```python
from build123d import *

# Parameters (mm, degrees)
BOSS_EXTRUDE1_DEPTH = 12.7
SKETCH1_10_R        = 3.175
SKETCH1_10_R_2      = 6.35
CUT_EXTRUDE3_DEPTH  = 12.7
SKETCH2_W           = 2.54
SKETCH2_H           = 25.4
CUT_EXTRUDE4_DEPTH  = 10.16
SKETCH2_3_W         = 20.32
SKETCH2_3_H         = 3.81
BOSS_EXTRUDE2_DEPTH = 10.16


with BuildPart() as part:
    # Sketch1 → Boss-Extrude1 (new, symmetric)
    with BuildSketch(Plane.XY):
        with BuildLine():
            Line((609.6, 0), (609.6, 25.4))
            Line((609.6, 25.4), (76.2, 25.4))
            ThreePointArc((76.2, 25.4), (63.5, 12.7), (76.2, 0))
            Line((76.2, 0), (609.6, 0))
        make_face()
    extrude(amount=BOSS_EXTRUDE1_DEPTH, both=True)

    # Sketch1<10> → Cut-Extrude3 (cut, symmetric)
    with BuildSketch(Plane.XY):
        with Locations((76.2, 12.7)):
            Circle(SKETCH1_10_R)
        with Locations((139.699994312, 12.7)):
            Circle(SKETCH1_10_R_2)
    extrude(amount=CUT_EXTRUDE3_DEPTH, both=True, mode=Mode.SUBTRACT)

    # Sketch2 → Cut-Extrude4 (cut)
    with BuildSketch(Plane(origin=(609.6, 0, 0), x_dir=(0, 0, -1), z_dir=(1, 0, 0))):
        with Locations((-11.43, 12.7)):
            Rectangle(SKETCH2_W, SKETCH2_H)
        with Locations((11.43, 12.7)):
            Rectangle(SKETCH2_W, SKETCH2_H)
    extrude(amount=-CUT_EXTRUDE4_DEPTH, mode=Mode.SUBTRACT)

    # Sketch2<3> → Boss-Extrude2 (add)
    with BuildSketch(Plane(origin=(609.6, 0, 0), x_dir=(0, 0, -1), z_dir=(1, 0, 0))):
        with Locations((0, 27.305)):
            Rectangle(SKETCH2_3_W, SKETCH2_3_H)
        with Locations((0, -1.905)):
            Rectangle(SKETCH2_3_W, SKETCH2_3_H)
    extrude(amount=-BOSS_EXTRUDE2_DEPTH)


solid = part.part
```
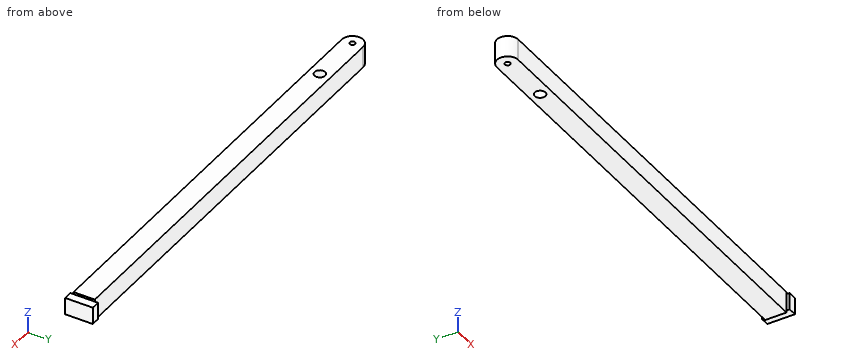
Here's how the part is built. I have some questions about the finished solid (model axes, mm). Give positions to 0.01 mm unless a question says otherwise; leave off trailing zeros. Write each loop counter-clockwise with the first axis right and the second up, starting at its lowest first coordinate (ties: lowest second). Pieces come first, ordered by that corner, then holes. Notation, with made-up numbers: M 0,-1.75 L 10,-1.75 A19 ccw 10,11.25 Z; hole C -39.5,41.25 d9. An arc over 180 degrees is marked long. Put each result on its own line as item: value. Start each with the question number.
Item 1: Will these pins go through, and if not, where does the flat tip stop? pin 1 (7.5 mm diameter, centred on x = 376.5, z = -6, fed in from -Y); pin 2 (11 mm diameter, centred on x = 605, y = 15.5, fed in from -Z); pin 3 (3 mm diameter, centred on y = 10.5, z = -12, fed in from +X).
Item 2: I need wall thicknesses on L1, parallel to X at y = 13, z = -6.25; L2, parallel to Y at x = 76.2, z = 7.25 (3 decimals); L3, parallel to X at y = 15, z = 2.5. Which ranges of each line are inside material? Lowest first, please. Write a range as from..to.
Item 3: If we section it at A-A, the plane z = -0.5: Write out the boundary of the cut face in (x, y) (3 decimals), then the cut area to 3 significant figures.
Item 4: If we section it at B-B, the plane x = 461: Write out the boundary of the cut face in (y, z).
Values:
1. pin 1: y = 0
1. pin 2: z = -10.16
1. pin 3: x = 599.44
2. L1: 63.5..73.04, 79.36..133.36, 146.04..609.6
2. L2: 0..9.525, 15.875..25.4
2. L3: 63.71..74.01, 78.39..133.78, 145.62..609.6
3. outline: M 76.2,0 L 599.44,0 L 599.44,-3.81 L 609.6,-3.81 L 609.6,29.21 L 599.44,29.21 L 599.44,25.4 L 76.2,25.4 A12.7 ccw Z; hole C 76.2,12.7 d6.35; hole C 139.7,12.7 d12.7
3. area: 13,700 mm²
4. outline: M 0,-12.7 L 25.4,-12.7 L 25.4,12.7 L 0,12.7 Z
